```python
from build123d import *
from OCP.BRepFilletAPI import BRepFilletAPI_MakeChamfer

# Parameters (mm, degrees)
SKETCH1_W           = 1350
SKETCH1_H           = 250
BOSS_EXTRUDE1_DEPTH = 70
CHAMFER1_SIZE       = 10
CHAMFER1_SIZE2      = 20
SHELL1_T            = 10
SKETCH2_W           = 30
SKETCH2_H           = 250
BOSS_EXTRUDE2_DEPTH = 25
CHAMFER2_SIZE       = 20
FILLET1_R           = 10
SKETCH3_R           = 10
BOSS_EXTRUDE3_DEPTH = 25
CHAMFER3_SIZE       = 3


with BuildPart() as part:
    # Sketch1 → Boss-Extrude1 (new body)
    with BuildSketch(Plane(origin=(0, 0, 0), x_dir=(1, 0, 0), z_dir=(0, 1, 0))):
        Rectangle(SKETCH1_W, SKETCH1_H)
    extrude(amount=BOSS_EXTRUDE1_DEPTH)

    # Chamfer1: one chamfer whose edges measure the first distance from different faces: ONE call of the kernel's chamfer builder (chamfer() names one face for all edges)
    chamfer1_edges_1 = [part.edges().sort_by_distance(p)[0] for p in [
        (675, 70, 0),
    ]]
    chamfer1_side_1 = [part.faces().sort_by_distance(p)[0] for p in [
        (675, 35, 0),
    ]]
    chamfer1_edges_2 = [part.edges().sort_by_distance(p)[0] for p in [
        (0, 70, -125),
    ]]
    chamfer1_side_2 = [part.faces().sort_by_distance(p)[0] for p in [
        (0, 35, -125),
    ]]
    chamfer1_edges_3 = [part.edges().sort_by_distance(p)[0] for p in [
        (-675, 70, 0),
    ]]
    chamfer1_side_3 = [part.faces().sort_by_distance(p)[0] for p in [
        (-675, 35, 0),
    ]]
    chamfer1_edges_4 = [part.edges().sort_by_distance(p)[0] for p in [
        (0, 70, 125),
    ]]
    chamfer1_side_4 = [part.faces().sort_by_distance(p)[0] for p in [
        (0, 35, 125),
    ]]
    chamfer1 = BRepFilletAPI_MakeChamfer(part.part.solid().wrapped)
    for e in chamfer1_edges_1:
        chamfer1.Add(CHAMFER1_SIZE, CHAMFER1_SIZE2, e.wrapped, chamfer1_side_1[0].wrapped)  # the first distance lies on this face
    for e in chamfer1_edges_2:
        chamfer1.Add(CHAMFER1_SIZE, CHAMFER1_SIZE2, e.wrapped, chamfer1_side_2[0].wrapped)  # the first distance lies on this face
    for e in chamfer1_edges_3:
        chamfer1.Add(CHAMFER1_SIZE, CHAMFER1_SIZE2, e.wrapped, chamfer1_side_3[0].wrapped)  # the first distance lies on this face
    for e in chamfer1_edges_4:
        chamfer1.Add(CHAMFER1_SIZE, CHAMFER1_SIZE2, e.wrapped, chamfer1_side_4[0].wrapped)  # the first distance lies on this face
    add(Compound.cast(chamfer1.Shape()), mode=Mode.REPLACE)

    # Shell1 (no face opened: a closed hollow body)
    add(offset(amount=-SHELL1_T, mode=Mode.PRIVATE), mode=Mode.SUBTRACT)

    # Sketch2 → Boss-Extrude2 (add)
    with BuildSketch(Plane.XZ):
        with Locations((-90, 0)):
            Rectangle(SKETCH2_W, SKETCH2_H)
        with Locations((90, 0)):
            Rectangle(SKETCH2_W, SKETCH2_H)
    extrude(amount=BOSS_EXTRUDE2_DEPTH)

    # Chamfer2
    chamfer2_edges = [part.edges().sort_by_distance(p)[0] for p in [
        (-105, 0, 0),
        (105, 0, 0),
    ]]
    chamfer(chamfer2_edges, length=CHAMFER2_SIZE)

    # Fillet1
    fillet1_edges = [part.edges().sort_by_distance(p)[0] for p in [
        (-400, 0, -125),
        (675, 0, 0),
        (-400, 0, 125),
        (-675, 0, 0),
        (-125, 0, 0),
        (400, 0, -125),
        (400, 0, 125),
        (125, 0, 0),
        (-115, -10, -125),
        (-115, -10, 125),
        (115, -10, 125),
        (115, -10, -125),
    ]]
    fillet(fillet1_edges, radius=FILLET1_R)

    # Sketch3 → Boss-Extrude3 (add)
    with BuildSketch(Plane.XZ):
        with Locations(Location((0, 0, 0), (0, 0, 90))):
            Circle(SKETCH3_R)
    extrude(amount=BOSS_EXTRUDE3_DEPTH)

    # Chamfer3
    chamfer3_edges = [part.edges().sort_by_distance(p)[0] for p in [
        (0, -25, -10),
    ]]
    chamfer(chamfer3_edges, length=CHAMFER3_SIZE)


solid = part.part
```
The model under review builds one solid part; all positions refer to its coordinate system, in mm. A direction names the side the tool comes from. Round coordinates to 2 decimals unless told otherwise and drop trailing zeros. Loops run counter-clockwise (first coordinate to the right, second up) from the corner with the lowest first, then second, coordinate; pieces in that order, holes last.
1) Clearance check with flat-ended pins moving along their axes: P1, Ø12.5, axis at y = -8.5, z = -21.5, coming from the +X side; P2, Ø6, axis at x = 253, y = 1.5, coming from the -Z side; P3, Ø9.5, axis at y = -18.5, z = 41, coming from the +X side. State where each tip first meets the part, or that it passes through.
Values follow:
P1: stops at x = 122.82
P2: stops at z = -123.35
P3: stops at x = 111.25
2) Consider section C-C on y = 39.5. State the section outline as (x, z) points, then the cut area to 3 significant figures.
Values follow:
outline: (-675, -125) - (675, -125) - (675, 125) - (-675, 125) - close; hole (-665, -115) - (665, -115) - (665, 115) - (-665, 115) - close
area: 31,600 mm2
3) The part is to be moulded in two halves that separate along X. For faces 1 (the face through (75, -12, -2)), 2 (the face through (-75, -12, -2)), 3 (the face through (90, -25, 2)), 4 (the face through (-675, 35, 2)), say which applies: pulls with the +X half, pulls with the -X half, needs draft (parallel to the pull), parting line crosses it, or undercut.
Values follow:
face 1: undercut
face 2: undercut
face 3: needs draft
face 4: pulls with the -X half
4) Wall thickness on line 1 along Y through (x, z) = (377, -3); line 2 along X through (y, z) = (47.5, 38); line 3 along Z through (x, y) = (-300.5, 19.5): over which ranges is each line inside the solid? List them lowest first.
Values follow:
line 1: y = 0 to 10, 60 to 70
line 2: x = -675 to -665, 665 to 675
line 3: z = -125 to -115, 115 to 125
5) Tool access review of faces 5 (the face through (-9, 70, -1)), 6 (the face through (-401, 0, -2)), 7 (the face through (393, 0, -2)), 8 (the face through (-665, 32, 2)), 9 (the face through (-9, 36, -125)): name each direction out of +Z, -Z, +X, -X, +Y, -Y from which nothing blocks a thin tool from reaching the whole face with its end or side.
Values follow:
face 5: +Z, -Z, +X, -X, +Y
face 6: +Z, -Z, -X, -Y
face 7: +Z, -Z, +X, -Y
face 8: none
face 9: -Z, +X, -X, +Y, -Y
6) Consider section B-B on x = -589. State the section outline as (y, z) points.
Values follow:
outline: (0, -115) arc R10 ccw to (10, -125) - (60, -125) - (70, -105) - (70, 105) - (60, 125) - (10, 125) arc R10 ccw to (0, 115) - close; hole (10, -115) - (53.82, -115) - (60, -102.64) - (60, 102.64) - (53.82, 115) - (10, 115) - close
7) Consider section A-A on z = -62. State the section outline as (x, y) points, then the cut area to 3 significant figures.
Values follow:
outline: (-675, 10) arc R10 ccw to (-665, 0) - (-129.14, 0) arc R10 cw to (-122.07, -2.93) - (-105, -20) - (-105, -25) - (-75, -25) - (-75, 0) - (75, 0) - (75, -25) - (105, -25) - (105, -20) - (122.07, -2.93) arc R10 cw to (129.14, 0) - (665, 0) arc R10 ccw to (675, 10) - (675, 60) - (655, 70) - (-655, 70) - (-675, 60) - close; hole (-665, 10) - (665, 10) - (665, 53.82) - (652.64, 60) - (-652.64, 60) - (-665, 53.82) - close
area: 29,700 mm2
